Verification items for the finished model (mm, model axes). A direction names the side the tool comes from. Round coordinates to 2 decimals unless told otherwise and drop trailing zeros. Write each loop counter-clockwise with the first axis right and the second up, starting at its lowest first coordinate (ties: lowest second). Pieces come first, ordered by that corner, then holes. Notation, with made-up numbers: M 40.5,20 L 63.5,20 A3 cw 63.5,25 Z; hole C 27.5,61 d8. An arc over 180 degrees is marked long. Use a Markdown table: item, result. Add a question column.
Autodesk Inventor part; units mm, degrees
ref_plane "YZ Plane" through (0, 0, 0) normal (1, 0, 0) x (0, 1, 0)
ref_plane "XZ Plane" through (0, 0, 0) normal (0, 1, 0) x (-1, 0, 0)
ref_plane "XY Plane" through (0, 0, 0) normal (0, 0, 1) x (1, 0, 0)
sketch "Эскиз1" plane through (0, 0, 0) normal (0, 1, 0) x (-1, 0, 0)
  line L0 (0, 0) -> (0, -12)
  line L1 (0, -12) -> (0, -20)
  line L2 (-5, -15) -> (5, -15)
  line L3 (5, -15) -> (5, -25)
  line L4 (5, -25) -> (-5, -25)
  line L5 (-5, -25) -> (-5, -15)
  line L6 (-5, -15) -> (5, -25) construction
  line L7 (5, -15) -> (-5, -25) construction
  circle A0 centre (0, -20) radius 1.5
  dimension "d0" = 12
  dimension "d1" = 8
  dimension "d2" = 10
  dimension "d3" = 10
  dimension "d4" = 3
extrude "Выдавливание1" add sketch "Эскиз1" along normal blind 3
sketch "Эскиз2" plane through (0, 3, 0) normal (0, 1, 0) x (1, 0, 0)
  line L0 (-5, 15) -> (5, 15)
  line L1 (-5, 15) -> (5, 15)
  line L2 (5, 15) -> (5, 12)
  line L3 (5, 12) -> (-5, 12)
  line L4 (-5, 12) -> (-5, 15)
  point P0 (0, 0)
  dimension "d7" = 3
extrude "Выдавливание2" add sketch "Эскиз2" along normal blind 7.2 and the other way blind 3
sketch "Эскиз3" plane through (0, 10.2, 0) normal (0, 1, 0) x (1, 0, 0)
  line L0 (5, 15) -> (-5, 15)
  line L1 (5, 15) -> (-5, 15)
  line L2 (-5, 15) -> (-5, 0)
  line L3 (-5, 0) -> (5, 0)
  line L4 (5, 0) -> (5, 15)
  point P0 (0, 0)
  dimension "d12" = 10
extrude "Выдавливание3" add sketch "Эскиз3" along normal blind 3
mirror "Зеркальное отражение1" about plane through (0, 0, 0) normal (0, 0, 1) of "Выдавливание2", "Выдавливание3", "Выдавливание1"
properties part number "000.210 - Скоба"
1. Cross-section at D-D on x = -3.75. Enter the section's corners in (y, z).
2. Depth check by flat-ended pin: pin 1 Ø3 at (x, y) = (-0.5, 6.5) entering from -Z; pin 2 Ø5 at (x, z) = (1, 21.5) entering from +Y; pin 3 Ø3 at (x, y) = (1, 7.5) entering from +Z; pin 4 Ø2.5 at (x, z) = (0, 20) entering from -Y. Enter the tip coordinate at first touch or a pass-through.
3. Release check for a two-part mould opening along X. For faces 5 (the flat face through (-5, 11, 2)), 6 (the cylindrical face through (0.195, 1.479, -21.487)), 7 (the flat face through (0, 0, 18)) record: +X half, -X half, draft (parallel to the pull), parting line (faces both ways), or undercut.
4. Access from +Z, -Z, +X, -X, +Y, -Y to the whole of each face (thin tool, end or side, straight path). Record for faces 1 (the flat face through (0, 8, 15)), 2 (the flat face through (0, 5, -12)), 3 (the flat face through (1.2, 3, -18.8)), 4 (the flat face through (5, 11, -2)).
5. Cross-section at A-A on x = 0. Enter the section's corners in (y, z), plus the area to 3 significant figures.
6. Cross-section at C-C on z = 20. Enter the section's corners in (x, y), plus the area to 3 significant figures.
7. Scan lines: line 1 along Z through (x, y) = (0, 0.6); line 2 along Z through (x, y) = (3.25, 6.5); line 3 along Z through (x, y) = (-3.5, 1). Record each from-to range of solid material in increasing order. Write a range as from..to.
8. Cross-section at B-B on y = 2. Enter the section's corners in (x, z), plus the area to 3 significant figures.
Answer:
| question | item | result |
|---|---|---|
| 1 | outline | M 0,-25 L 3,-25 L 3,-15 L 13.2,-15 L 13.2,15 L 3,15 L 3,25 L 0,25 L 0,12 L 10.2,12 L 10.2,-12 L 0,-12 Z |
| 2 | pin 1 | stops at z = -15 |
| 2 | pin 2 | stops at y = 3 |
| 2 | pin 3 | stops at z = 15 |
| 2 | pin 4 | passes through |
| 3 | face 5 | -X half |
| 3 | face 6 | undercut |
| 3 | face 7 | draft |
| 4 | face 1 | +Z, +X, -X, +Y |
| 4 | face 2 | +X, -X, -Y |
| 4 | face 3 | -Z, +X, -X, +Y |
| 4 | face 4 | +Z, -Z, +X, +Y, -Y |
| 5 | outline | M 0,-25 L 3,-25 L 3,-21.5 L 0,-21.5 Z; M 0,-18.5 L 3,-18.5 L 3,-15 L 13.2,-15 L 13.2,15 L 3,15 L 3,18.5 L 0,18.5 L 0,12 L 10.2,12 L 10.2,-12 L 0,-12 Z; M 0,21.5 L 3,21.5 L 3,25 L 0,25 Z |
| 5 | area | 193 mm^2 |
| 6 | outline | M -5,0 L -1.5,0 L -1.5,3 L -5,3 Z; M 1.5,0 L 5,0 L 5,3 L 1.5,3 Z |
| 6 | area | 21.0 mm^2 |
| 7 | line 1 | z = -25..-21.5, -18.5..-12, 12..18.5, 21.5..25 |
| 7 | line 2 | z = -15..-12, 12..15 |
| 7 | line 3 | z = -25..-12, 12..25 |
| 8 | outline | M -5,-25 L 5,-25 L 5,-12 L -5,-12 Z; M -5,12 L 5,12 L 5,25 L -5,25 Z; hole C 0,-20 d3; hole C 0,20 d3 |
| 8 | area | 246 mm^2 |
